```python
from build123d import *

# Parameters (mm, degrees)
PAD_DEPTH     = 8
SKETCH002_R   = 7
PAD001_DEPTH  = 4.5
POCKET_DEPTH  = 5
SKETCH005_R   = 6
SKETCH005_R_2 = 2.6
PAD002_DEPTH  = 10


with BuildPart() as part:
    # Sketch001 → Pad (new body, symmetric)
    with BuildSketch(Plane.XY):
        with BuildLine():
            ThreePointArc((-37.080992, 65), (-7.64069, 10.736533), (40, 50))
            Line((40, 50), (50, 50))
            ThreePointArc((-47.69696, 65), (-7.587885, 0.579114), (50, 50))
            Line((-47.69696, 65), (-37.080992, 65))
        make_face()
    extrude(amount=PAD_DEPTH, both=True)

    # Sketch002 → Pad001 (join, symmetric)
    with BuildSketch(Plane.XZ):
        Circle(SKETCH002_R)
    extrude(amount=PAD001_DEPTH, both=True)

    # Sketch004 (on Face8 of Pad001) → Pocket (cut)
    with BuildSketch(Plane.XZ.offset(4.5)):
        with BuildLine():
            Line((-1.532971, 2.1), (1.532971, 2.1))
            ThreePointArc((1.532971, -2.1), (2.6, 0), (1.532971, 2.1))
            Line((-1.532971, -2.1), (1.532971, -2.1))
            ThreePointArc((-1.532971, 2.1), (-2.6, 0), (-1.532971, -2.1))
        make_face()
    extrude(amount=-POCKET_DEPTH, mode=Mode.SUBTRACT)

    # Sketch005 (on Face8 of Pocket) → Pad002 (join)
    with BuildSketch(Plane.XZ.offset(4.5)):
        Circle(SKETCH005_R)
        Circle(SKETCH005_R_2, mode=Mode.SUBTRACT)
    extrude(amount=PAD002_DEPTH)


solid = part.part
```
The model under review builds one solid part; all positions refer to its coordinate system, in mm. A direction names the side the tool comes from. Round coordinates to 2 decimals unless told otherwise and drop trailing zeros. Order: outer loops, then holes, each group sorted by start corner. A loop starts at its lowest first (then second) coordinate and runs counter-clockwise, first axis right, second up. Notation, with made-up numbers: (64, 27.5) -> (101, 27.5) arc R21 ccw to (101, 49.5) -> close; hole circle Ø4 at (33, 35). An arc over 180 degrees is marked (long way). One line per item, written item: value. Start each with the question number.
Q1. Clearance check with flat-ended pins moving along their axes: pin 1 Ø2.5 at (x, y) = (-0.5, -2.5) entering from -Z; pin 2 Ø1 at (x, z) = (-7, 5.5) entering from +Y; pin 3 Ø4.5 at (x, z) = (0, -0.5) entering from -Y; pin 4 Ø1.5 at (x, z) = (-24, 3.5) entering from +Y. State where each tip first meets the part, or that it passes through.
Q2. Take a section at B-B (x = 0). Write out the cut boundary in (y, z).
Q3. Machinability: for faces 1 (the face through (-42, 65, 0)), 2 (the face through (-7, -2, 0)), 3 (the face through (45, 50, 0)), which of the approach directions +Z, -Z, +X, -X, +Y, -Y give a long, thin tool a straight path to every point of the face, cutting with its end or side? Answer none if there is none.
Q4. Mouldability with a two-part tool opening along X and no side actions: class faces 4 (the face through (-11, 11, 8)), 5 (the face through (0, -2, 2.1)), 6 (the face through (-6, -9, 0)), 7 (the face through (0, 0.5, 0)) as released by +X, released by -X, zero draft, split by the parting line, or undercut.
Q5. Take a section at D-D (y = 3.5). Write out the cut boundary in (x, z).
Q6. Take a section at C-C (z = -4.25). Write out the cut boundary in (x, y), and give its area (3 significant figures).
Q7. Take a section at A-A (y = 26). Write out the cut boundary in (x, z), and give its area (3 significant figures).
Q8. Wall thickness on line 1 (X direction, y = -2.5, z = 0); line 2 (X direction, y = 15.5, z = 6.25); line 3 (Z direction, x = 0, y = -6): over which ranges is each line inside the solid? List them lowest first.
Reported:
1. pin 1: stops at z = -7
1. pin 2: stops at y = 10.71
1. pin 3: stops at y = -14.5
1. pin 4: stops at y = 18.58
2. outline: (-14.5, -6) -> (-4.5, -6) -> (-4.5, -7) -> (0, -7) -> (0, -8) -> (10, -8) -> (10, 8) -> (0, 8) -> (0, 7) -> (-4.5, 7) -> (-4.5, 6) -> (-14.5, 6) -> (-14.5, 2.6) -> (-4.5, 2.6) -> (-4.5, 2.1) -> (0.5, 2.1) -> (0.5, -2.1) -> (-4.5, -2.1) -> (-4.5, -2.6) -> (-14.5, -2.6) -> close
3. face 1: +Z, -Z, +X, -X, +Y
3. face 2: -Y
3. face 3: +Z, -Z, +X, +Y
4. face 4: zero draft
4. face 5: undercut
4. face 6: split by the parting line
4. face 7: undercut
5. outline: (-18.38, -8) -> (18.38, -8) -> (18.38, 8) -> (-18.38, 8) -> close
6. outline: (-47.7, 65) arc R50 ccw to (-5.56, 0.31) -> (-5.56, -4.5) -> (-4.24, -4.5) -> (-4.24, -14.5) -> (4.24, -14.5) -> (4.24, -4.5) -> (5.56, -4.5) -> (5.56, 0.31) arc R50 ccw to (50, 50) -> (40, 50) arc R40 cw (long way) to (-37.08, 65) -> close
6. area: 1,700 mm2
7. outline: (-43.86, -8) -> (-32, -8) -> (-32, 8) -> (-43.86, 8) -> close; (32, -8) -> (43.86, -8) -> (43.86, 8) -> (32, 8) -> close
7. area: 380 mm2
8. line 1: x = -7 to -2.6, 2.6 to 7
8. line 2: x = -36.19 to -20.24, 20.24 to 36.19
8. line 3: z = -6 to -2.6, 2.6 to 6
